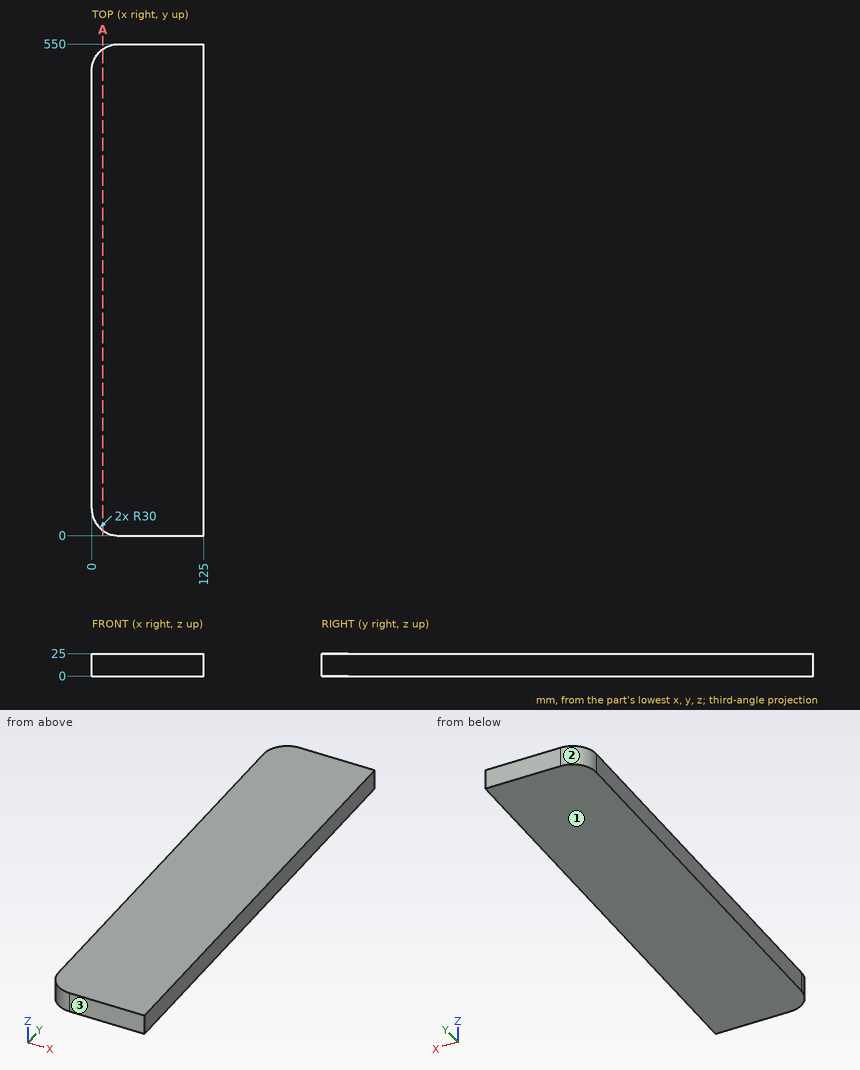
Job drawing, mm, ordinate dimensions from the low corner. One solid piece. Give positions to 0.01 mm unless a question says otherwise; leave off trailing zeros. Loops run counter-clockwise (first coordinate to the right, second up) from the corner with the lowest first, then second, coordinate; pieces in that order, holes last. Notation, with made-up numbers: M -38.75,78 L -32.75,78 A14 ccw -32.75,92 Z; hole C 30,12.25 d3. An arc over 180 degrees is marked long. Use one line per item in the form item = value.
Item 1: Slice it at A-A on x = 12.5. List the corners of the cut face in (y, z).
Filled in:
outline = M 5.63,0 L 544.37,0 L 544.37,25 L 5.63,25 Z
Item 2: Drill centre lines: L1, parallel to Y at x = 9, z = 2.75; L2, parallel to Y at x = 10.5, z = 22. Where is each one in solid material? Low to high.
Filled in:
L1 = 8.58 to 541.42
L2 = 7.2 to 542.8
Item 3: Two-plate mould, pull along Y, no slides. Class the marked faces 1, 2 and 3: released by +Y, released by -Y, zero draft, split by the parting line, or undercut.
Filled in:
face_1 = zero draft
face_2 = released by +Y
face_3 = released by -Y
